Autodesk Inventor part; units mm, degrees
ref_plane "YZ Plane" through (0, 0, 0) normal (1, 0, 0) x (0, 1, 0)
ref_plane "XZ Plane" through (0, 0, 0) normal (0, 1, 0) x (-1, 0, 0)
ref_plane "XY Plane" through (0, 0, 0) normal (0, 0, 1) x (1, 0, 0)
sketch "Sketch2" plane through (0, 0, 0) normal (0, 1, 0) x (-1, 0, 0)
  line L0 (38.4103, 71.1381) -> (-0.4517, 71.1381)
  line L1 (-0.4517, 71.1381) -> (-0.4517, -9.3799)
  line L2 (-0.4517, -9.3799) -> (38.4103, -9.3799)
  line L3 (38.4103, -9.3799) -> (38.4103, 71.1381)
  point P0 (0, 0)
  dimension "d0" = 38.862
  dimension "d1" = 80.518
extrude "Extrusion1" add sketch "Sketch2" along normal blind 25.4
fillet "Fillet1" radius 3.175 4 edges at (-38.4103, 12.7, -9.3799) (0.4517, 12.7, -9.3799) (-38.4103, 12.7, 71.1381) (0.4517, 12.7, 71.1381)
sketch "Sketch3" plane through (0, 0, 0) normal (0, -1, 0) x (1, 0, 0)
  line L0 (-7.1683, 61.3591) -> (-30.7903, 61.3591)
  line L1 (-30.7903, 61.3591) -> (-30.7903, 0.3991)
  line L2 (-30.7903, 0.3991) -> (-7.1683, 0.3991)
  line L3 (-7.1683, 0.3991) -> (-7.1683, 61.3591)
  line L4 (-38.4103, -6.2049) -> (-38.4103, 67.9631)
  line L5 (-30.7903, 30.8791) -> (-38.4103, 30.8791) construction
  line L6 (-2.7233, -9.3799) -> (-35.2353, -9.3799) construction
  line L7 (-18.9793, 0.3991) -> (-18.9793, -9.3799) construction
  line L8 (-7.1683, 30.8791) -> (0.4517, 30.8791) construction
  line L9 (0.4517, 67.9631) -> (0.4517, -6.2049) construction
  line L10 (-18.9793, 61.3591) -> (-18.9793, 71.1381) construction
  line L11 (-35.2353, 71.1381) -> (-2.7233, 71.1381) construction
  point P0 (0, 0)
  dimension "d5" = 23.622
  dimension "d6" = 60.96
extrude "Extrusion2" cut sketch "Sketch3" against normal blind 2.54
fillet "Fillet2" radius 1.524 4 edges at (-30.7903, 1.27, 61.3591) (-30.7903, 1.27, 0.3991) (-7.1683, 1.27, 61.3591) (-7.1683, 1.27, 0.3991)
sketch "Sketch4" plane through (0.0246, 25.4, 6.6784) normal (0, 1, 0) x (1, 0, 0)
  line L0 (-2.8421, -22.9344) -> (-9.1921, -22.9344)
  line L1 (-9.1921, -22.9344) -> (-9.1921, -41.9844)
  line L2 (-9.1921, -41.9844) -> (-2.8421, -41.9844)
  line L3 (-2.8421, -41.9844) -> (-2.8421, -22.9344)
  point P0 (0, 0)
  dimension "d10" = 6.35
  dimension "d11" = 19.05
extrude "Extrusion3" cut sketch "Sketch4" against normal blind 2.54
fillet "Fillet3" radius 1.27 4 edges at (-9.1674, 24.13, 29.6127) (-2.8174, 24.13, 29.6127) (-9.1674, 24.13, 48.6627) (-2.8174, 24.13, 48.6627)
sketch "Sketch6" plane through (0.0246, 22.86, 6.6784) normal (0, 1, 0) x (1, 0, 0)
  line L0 (-7.8199, -3.1416) -> (-4.0099, -3.1416)
  line L1 (-4.0099, -3.1416) -> (-4.0099, 0.6684)
  line L2 (-4.0099, 0.6684) -> (-7.8199, 0.6684)
  line L3 (-7.8199, 0.6684) -> (-7.8199, -3.1416)
  line L4 (-7.8199, 6.6784) -> (-4.0099, 6.6784)
  line L5 (-4.0099, 6.6784) -> (-4.0099, 10.4884)
  line L6 (-4.0099, 10.4884) -> (-7.8199, 10.4884)
  line L7 (-7.8199, 10.4884) -> (-7.8199, 6.6784)
  point P0 (-0.0246, 6.6784)
  dimension "d16" = 3.81
  dimension "d17" = 3.81
  dimension "d18" = 3.81
  dimension "d19" = 3.81
extrude "Extrusion4" add sketch "Sketch6" along normal blind 2.54
extrude "Extrusion5" [suppressed]
sketch "Sketch8" plane through (-38.4103, 0, -6.2049) normal (-1, 0, 0) x (0, 0, 1)
  point P0 (6.2049, 0)
sketch "Sketch9" plane through (-38.4103, 0, -6.2049) normal (-1, 0, 0) x (0, 0, 1)
  point P0 (6.2049, 0)
sketch "Sketch10" plane through (-38.4103, 0, -6.2049) normal (-1, 0, 0) x (0, 0, 1)
  line L0 (74.168, 25.4) -> (74.168, 0)
  line L1 (0, 0) -> (0, 25.4)
  line L2 (74.168, 18.7302) -> (0, 18.7302)
  line L3 (0, 18.7302) -> (0, 6.0302)
  line L4 (0, 6.0302) -> (74.168, 6.0302)
  line L5 (74.168, 6.0302) -> (74.168, 18.7302)
  point P0 (6.2049, 0)
  dimension "d29" = 12.7
extrude "Extrusion6" cut sketch "Sketch10" against normal blind 10.16
fillet "Fillet4" radius 1.27 4 edges at (-33.3303, 18.7302, 67.9631) (-33.3303, 6.0302, 67.9631) (-33.3303, 18.7302, -6.2049) (-33.3303, 6.0302, -6.2049)
properties part number "Automoblox Body"
Here's how the part is built. I have some questions about the finished solid (model axes, mm). A direction names the side the tool comes from. Round coordinates to 2 decimals unless told otherwise and drop trailing zeros. Loops run counter-clockwise (first coordinate to the right, second up) from the corner with the lowest first, then second, coordinate; pieces in that order, holes last. Notation, with made-up numbers: (-13, 57.25) -> (27, 57.25) arc R6 cw to (27, 61.25) -> close; hole circle Ø3 at (-21, -14). An arc over 180 degrees is marked (long way). Answer as CSV lines item,"result". Start each with the question number.
1. Imagine slicing it at D-D on z = -0.5. Write out the boundary of the cut face in (x, y), plus the area to 3 significant figures.
2. I'm going to push flat-ended pins straight in: P1, Ø4, axis at y = 9.5, z = 24.5, coming from the -X side; P2, Ø3, axis at x = -6, z = 39, coming from the +Y side; P3, Ø6, axis at x = -17.5, z = 43, coming from the -Y side. Where does each tip first touch, or does it pass through?
3. Imagine slicing it at C-C on x = -23. Write out the boundary of the cut face in (y, z), plus the area to 3 significant figures.
4. Imagine slicing it at B-B on y = 10.5. Write out the boundary of the cut face in (x, z) (3 decimals), plus the area to 3 significant figures.
5. For faces 4 (the face through (-7.168, 1, 30)), 5 (the face through (-38.41, 22, 30)), 6 (the face through (-33, 18.73, 31)), 7 (the face through (-6, 24, 29.613)), 8 (the face through (-37.505, 12.878, 70.183)), which set-ups out of +Z, -Z, +X, -X, +Y, -Y let a thin tool reach every point of the face, with its end or its side?
6. Imagine slicing it at A-A on z = 58.5. Write out the boundary of the cut face in (x, y).
7. If we mould it in two halves opening along X, with no side actions, what happens to faces 1 (the face through (-33, 12, 67.963)), 2 (the face through (-19, 2.54, 31)), 3 (the face through (0.452, 13, 31))? For each: pulls with the +X half, pulls with the -X half, needs draft (parallel to the pull), parting line crosses it, or undercut.
8. I need wall thicknesses on probe 1 along Z at (x, y) = (-23.5, 1.25); probe 2 along X at (y, z) = (2.25, 19.5); probe 3 along Y at (x, z) = (-32.5, 45). Which ranges of each line are inside material? Lowest first, please. Write a range as from..to.
Solution:
1,outline,"(-38.41, 0) -> (0.45, 0) -> (0.45, 25.4) -> (-38.41, 25.4) -> (-38.41, 18.73) -> (-28.25, 18.73) -> (-28.25, 6.03) -> (-38.41, 6.03) -> close"
1,area,"858 mm²"
2,P1,"x = -28.25"
2,P2,"y = 22.86"
2,P3,"y = 2.54"
3,outline,"(0, -9.38) -> (25.4, -9.38) -> (25.4, 71.14) -> (0, 71.14) -> (0, 61.36) -> (2.54, 61.36) -> (2.54, 0.4) -> (0, 0.4) -> close"
3,area,"1,890 mm²"
4,outline,"(-38.41, -6.205) arc R3.175 ccw to (-35.235, -9.38) -> (-2.723, -9.38) arc R3.175 ccw to (0.452, -6.205) -> (0.452, 67.963) arc R3.175 ccw to (-2.723, 71.138) -> (-35.235, 71.138) arc R3.175 ccw to (-38.41, 67.963) -> (-28.25, 67.963) -> (-28.25, -6.205) -> close"
4,area,"2,370 mm²"
5,face 4,"-Y"
5,face 5,"+Z, -Z, -X, +Y, -Y"
5,face 6,"-X"
5,face 7,"+Y"
5,face 8,"+Z, -X, +Y, -Y"
6,outline,"(-38.41, 0) -> (-30.79, 0) -> (-30.79, 2.54) -> (-7.17, 2.54) -> (-7.17, 0) -> (0.45, 0) -> (0.45, 25.4) -> (-38.41, 25.4) -> (-38.41, 18.73) -> (-28.25, 18.73) -> (-28.25, 6.03) -> (-38.41, 6.03) -> close"
7,face 1,"needs draft"
7,face 2,"undercut"
7,face 3,"pulls with the +X half"
8,probe 1,"-9.38..0.4, 61.36..71.14"
8,probe 2,"-38.41..-30.79, -7.17..0.45"
8,probe 3,"0..6.03, 18.73..25.4"
